Answer from the drawing. Dimensions are ordinates in mm from the lowest x, y and z of the part. A direction names the side the tool comes from. Give positions to 0.01 mm unless a question says otherwise; leave off trailing zeros. Loops run counter-clockwise (first coordinate to the right, second up) from the corner with the lowest first, then second, coordinate; pieces in that order, holes last. Notation, with made-up numbers: (69.25, -32) - (94.25, -32) arc R37 cw to (94.25, 4) - close; hole circle Ø11 at (-11.75, 13.25). An arc over 180 degrees is marked (long way). One line per item, written item: value.
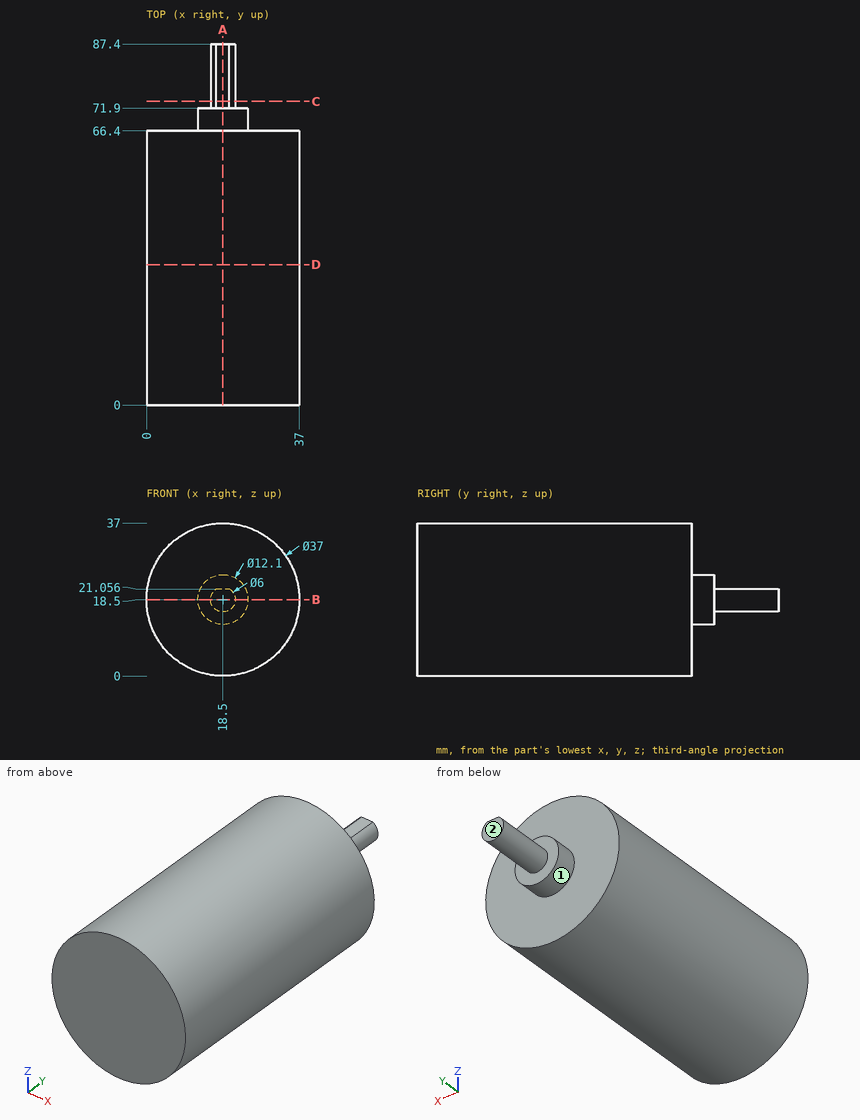
1. Flat-ended cylindrical pins translate along their axes: pin 1 Ø8 at (x, z) = (29.5, 6) entering from +Y; pin 2 Ø3 at (y, z) = (61.5, 23.5) entering from +X; pin 3 Ø6 at (x, z) = (23.5, 24) entering from +Y. Find the tip coordinate at first contact, or state that the pin passes through.
Output:
pin 1: stops at y = 66.4
pin 2: stops at x = 36.67
pin 3: stops at y = 71.9
2. Section A-A (x = 18.5) is taken. Write down the section's boundary in (y, z).
Output:
outline: (0, 0) - (66.4, 0) - (66.4, 12.45) - (71.9, 12.45) - (71.9, 15.5) - (87.4, 15.5) - (87.4, 21.06) - (71.9, 21.06) - (71.9, 24.55) - (66.4, 24.55) - (66.4, 37) - (0, 37) - close
3. Section D-D (y = 34) is taken. Write down the section's boundary in (x, z), and give its area (3 significant figures).
Output:
outline: circle Ø37 at (18.5, 18.5)
area: 1,080 mm²
4. For the marked faces 1 and 2, determine the directions among +Z, -Z, +X, -X, +Y, -Y from which every point of the face is accessible in a straight line to the end or side of a thin tool.
Output:
face 1: +Y
face 2: +Z, -Z, +X, -X, +Y
5. Section B-B (z = 18.5) is taken. Write down the section's boundary in (x, y).
Output:
outline: (0, 0) - (37, 0) - (37, 66.4) - (24.55, 66.4) - (24.55, 71.9) - (21.5, 71.9) - (21.5, 87.4) - (15.5, 87.4) - (15.5, 71.9) - (12.45, 71.9) - (12.45, 66.4) - (0, 66.4) - close
6. Find the intervals of material crossed by line 1 along Y through (x, z) = (17, 25); line 2 along Z through (x, y) = (19, 47); line 3 along Z through (x, y) = (15, 25.5) (1 decimal), in increasing order.
Output:
line 1: y = 0 to 66.4
line 2: z = 0.01 to 36.99
line 3: z = 0.3 to 36.7
7. Section C-C (y = 73.5) is taken. Write down the section's boundary in (x, z), and give its area (3 significant figures).
Output:
outline: (16.93, 21.06) arc R3 ccw (long way) to (20.07, 21.06) - close
area: 27.3 mm²
